For this review, take the finished solid that the model builds, in its own axes (mm). A direction names the side the tool comes from. Round coordinates to 2 decimals unless told otherwise and drop trailing zeros. Write each loop counter-clockwise with the first axis right and the second up, starting at its lowest first coordinate (ties: lowest second). Pieces come first, ordered by that corner, then holes. Notation, with made-up numbers: (14.25, 5) - (63.25, 5) arc R19 ccw to (63.25, 35) - close; hole circle Ø5 at (-34.5, -35). An arc over 180 degrees is marked (long way). One line per item, written item: value. Start each with the question number.
Q1. Tool access review of faces 3 (the face through (15, -7, -1)), 4 (the face through (1, 3, -10)), 5 (the face through (15, -7, 1)): name each direction out of +Z, -Z, +X, -X, +Y, -Y from which nothing blocks a thin tool from reaching the whole face with its end or side.
Q2. For probe 1 along Z at (x, y) = (13.5, -11); probe 2 along Y at (x, z) = (0, -2); probe 3 along Y at (x, z) = (2, -5.5), list the stretches that pass through material, from the lowest coordinate up.
Q3. Add section D-D on z = 5.75. Write out the cut boundary in (x, y).
Q4. Mouldability with a two-part tool opening along X and no side actions: class faces 1 (the face through (-3, 0, 0)), 2 (the face through (1, 3, 10)) as +X half, -X half, draft (parallel to the pull), parting line (faces both ways), or undercut.
Q5. Clearance check with flat-ended pins moving along their axes: pin 1 Ø4 at (y, z) = (-5, 8) entering from +X; pin 2 Ø8 at (x, y) = (0, 0) entering from -Z; pin 3 Ø3 at (x, y) = (-10, -15.5) entering from +Z; pin 4 Ø10 at (x, z) = (-4.5, 7) entering from +Y. State where each tip first meets the part, or that it passes through.
Q6. Add section C-C on z = -6. Write out the cut boundary in (x, y), and give its area (3 significant figures).
```python
from build123d import *

# Parameters (mm, degrees)
F0_R      = 4
F1_DEPTH  = 10
F2_R      = 35
F3_DEPTH  = 1
F6_R      = 0.99999
F7_R      = 3
F8_DEPTH  = 10.001
F9_R      = 3
F10_DEPTH = 10.001


# Not quite as in the source:
# - a fillet or chamfer that OpenCascade refuses, or shapes differently, is made with other operations: its cross-section is extruded or revolved along the edge and cut away or added
# - a fillet or chamfer is up to 0.001 mm smaller than in the source, because OpenCascade refuses the exact size


with BuildPart() as f1:
    # F0 (on Top) → F1 (new body, symmetric)
    with BuildSketch(Plane.XY):
        Circle(F0_R)
    extrude(amount=F1_DEPTH, both=True)

    # F2 (on Top) → F3 (join, symmetric)
    with BuildSketch(Plane.XY):
        Circle(F2_R)
    extrude(amount=F3_DEPTH, both=True)

    # F4: fillet of radius 12 on 1 edges, made by hand

    # F4_s1 → F4_t2 (revolve)
    with BuildSketch(Plane.XZ):
        with BuildLine():
            ThreePointArc((15.6189500386, 1), (8.2704808103, 3.5131670195), (4, 10))
            Line((4, 10), (4, 1))
            Line((4, 1), (15.6189500386, 1))
        make_face()
    revolve(axis=Axis((0, 0, 1), (0, 0, 1)))

    # F5: fillet of radius 12 on 1 edges, made by hand

    # F5_s1 → F5_t2 (revolve)
    with BuildSketch(Plane.XZ):
        with BuildLine():
            ThreePointArc((4, -10), (8.2704808103, -3.5131670195), (15.6189500386, -1))
            Line((15.6189500386, -1), (4, -1))
            Line((4, -1), (4, -10))
        make_face()
    revolve(axis=Axis((0, 0, -1), (0, 0, 1)))

    # F6 (radius 1 in the source; OpenCascade refuses exactly that, so slightly less here)
    f6_edges = [f1.edges().sort_by_distance(p)[0] for p in [
        (-35, 0, 1),
        (-35, 0, -1),
    ]]
    fillet(f6_edges, radius=F6_R)

    # F7 (on Top) → F8 (cut, through all)
    with BuildSketch(Plane.XY):
        Circle(F7_R)
    extrude(amount=-F8_DEPTH, mode=Mode.SUBTRACT)

    # F9 (on Top) → F10 (cut, through all)
    with BuildSketch(Plane.XY):
        Circle(F9_R)
    extrude(amount=F10_DEPTH, mode=Mode.SUBTRACT)


solid = f1.part
```
Result set:
1. face 3: -Z
1. face 4: -Z, +X, -X, +Y, -Y
1. face 5: +Z
2. probe 1: z = -1 to 1
2. probe 2: y = -10.82 to -3, 3 to 10.82
2. probe 3: y = -5.92 to -2.24, 2.24 to 5.92
3. outline: circle Ø12.11 at (0, 0); hole circle Ø6 at (0, 0)
4. face 1: undercut
4. face 2: draft
5. pin 1: stops at x = 4.14
5. pin 2: stops at z = -10
5. pin 3: stops at z = 1
5. pin 4: stops at y = 10.02
6. outline: circle Ø11.74 at (0, 0); hole circle Ø6 at (0, 0)
6. area: 80.1 mm^2
